```python
from build123d import *

# Parameters (mm, degrees)
F0_R     = 10
F0_R_2   = 2.5
F1_DEPTH = 25
F2_W     = 1
F2_H     = 1
F4_R     = 2
F5_R     = 4
F6_DEPTH = 20


with BuildPart() as f1:
    # F0 (on Front) → F1 (new body)
    with BuildSketch(Plane.XZ):
        Circle(F0_R)
        Circle(F0_R_2, mode=Mode.SUBTRACT)
    extrude(amount=-F1_DEPTH)

    # F2 (on Right) → F3 (revolve, cut)
    with BuildSketch(Plane.YZ):
        with Locations((11.5, 9.5)):
            Rectangle(F2_W, F2_H)
        with Locations((9.5, 9.5)):
            Rectangle(F2_W, F2_H)
        with Locations((13.5, 9.5)):
            Rectangle(F2_W, F2_H)
        with Locations((15.5, 9.5)):
            Rectangle(F2_W, F2_H)
    revolve(axis=Axis((0, 25, 0), (0, -1, 0)), mode=Mode.SUBTRACT)

    # F4
    f4_edges = [f1.edges().sort_by_distance(p)[0] for p in [
        (-10, 0, 0),
        (-10, 25, 0),
    ]]
    fillet(f4_edges, radius=F4_R)

    # F5 (on face) → F6 (cut)
    with BuildSketch(Plane.XZ):
        Circle(F5_R)
    extrude(amount=-F6_DEPTH, mode=Mode.SUBTRACT)


solid = f1.part
```
Geometry check sheet. Reference: the model listing, model coordinates, mm. A direction names the side the tool comes from. Round coordinates to 2 decimals unless told otherwise and drop trailing zeros. Order: outer loops, then holes, each group sorted by start corner. A loop starts at its lowest first (then second) coordinate and runs counter-clockwise, first axis right, second up. Notation, with made-up numbers: (-15.75, 52.25) - (27.25, 52.25) arc R14 cw to (27.25, 75.25) - close; hole circle Ø4 at (75, 23.5). An arc over 180 degrees is marked (long way). Use a Markdown table: item, result. Add a question column.
1) Section check A-A (y = 4.75). Record the cut outline in (x, z).
2) Set-up check for faces 4 (the cylindrical face through (-0.867, 9.86, -3.905)), 5 (the cylindrical face through (9.54, 14.49, 3)), 6 (the cylindrical face through (-8.923, 15.507, -1.172)): record each of +Z, -Z, +X, -X, +Y, -Y from which the full face is reachable in a straight line by a thin tool's end or side.
3) Gauge pin test, flat ends, axial feed: P1, Ø1, axis at x = -6.5, y = 5.5, coming from the -Z side; P2, Ø8, axis at x = -7.5, z = -4, coming from the +Y side; P3, Ø4, axis at y = 20.5, z = 4, coming from the +X side; P4, Ø1, axis at x = -5.5, y = 15, coming from the -Z side. Record the tip position at first contact, or that the pin passes through.
4) Mould release check, pull along Y, two halves, no side actions. Record for faces 1 (the flat face through (-4, 0, -2)), 2 (the cylindrical face through (-8.923, 11.507, -1.172)), 3 (the cylindrical face through (9.54, 5.45, 3)): released by +Y, released by -Y, zero draft, split by the parting line, or undercut.
5) Thickness scan on line 1 along Z through (x, y) = (0, 22.2); line 2 along Y through (x, z) = (1.5, 8); line 3 along X through (y, z) = (5.5, -3.25). Record the ranges inside material, lowest first.
6) Section check B-B (y = 9.5). Record the cut outline in (x, z).
Established:
| question | item | result |
|---|---|---|
| 1 | outline | circle Ø20 at (0, 0); hole circle Ø8 at (0, 0) |
| 2 | face 4 | -Y |
| 2 | face 5 | +Y, -Y |
| 2 | face 6 | none |
| 3 | P1 | z = -8 |
| 3 | P2 | y = 25 |
| 3 | P3 | x = 9.8 |
| 3 | P4 | z = -8.66 |
| 4 | face 1 | released by -Y |
| 4 | face 2 | undercut |
| 4 | face 3 | zero draft |
| 5 | line 1 | -10 to -2.5, 2.5 to 10 |
| 5 | line 2 | 0 to 25 |
| 5 | line 3 | -9.46 to -2.33, 2.33 to 9.46 |
| 6 | outline | circle Ø18 at (0, 0); hole circle Ø8 at (0, 0) |
